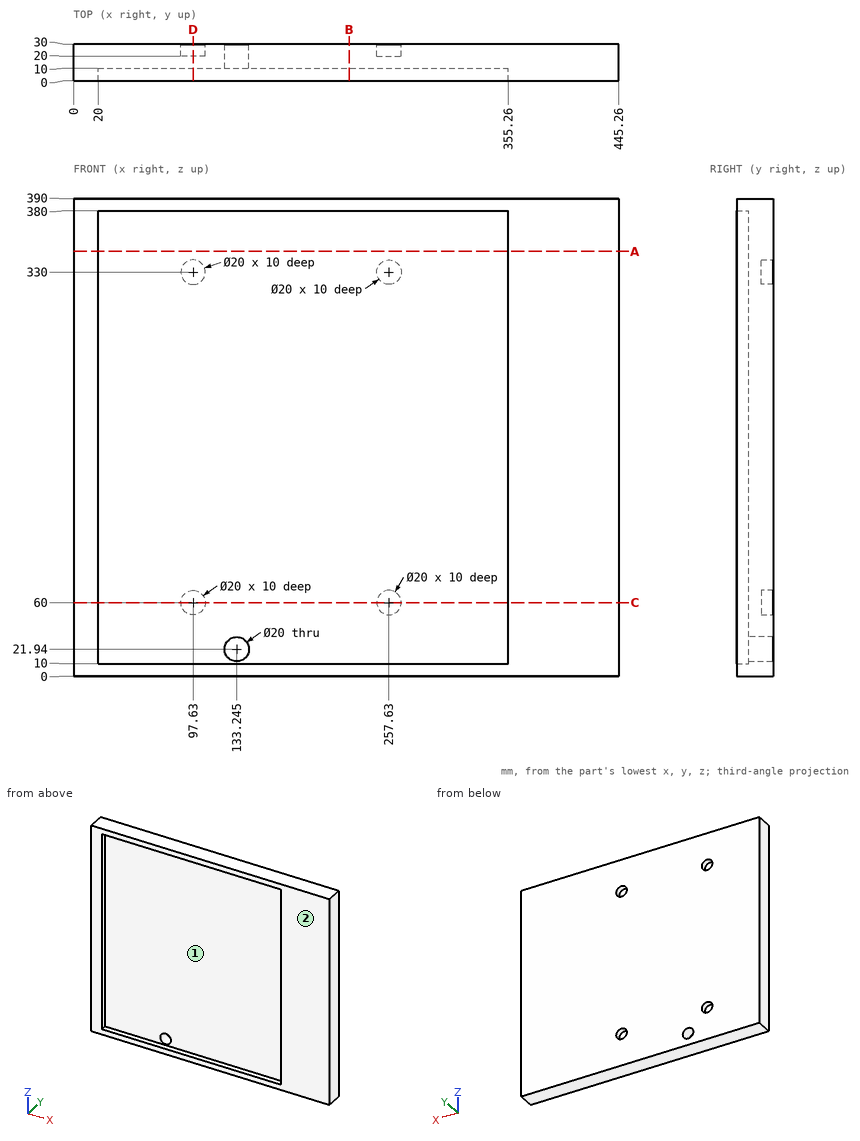
Geometry check sheet. Reference: drawing and pictorial views, mm from the part's lowest x, y, z. A direction names the side the tool comes from. Coordinates: 2 decimals unless noted, no trailing zeros. Write each loop counter-clockwise with the first axis right and the second up, starting at its lowest first coordinate (ties: lowest second). Pieces come first, ordered by that corner, then holes. Notation, with made-up numbers: M 21.5,28.5 L 60.5,28.5 A6 ccw 60.5,33.5 Z; hole C 86.5,10.5 d10. An arc over 180 degrees is marked long. Write item = value, one per line. Start each with the question number.
1. Sectioned sample at A-A (z = 347). Record the cut outline in (x, y), then the cut area to 3 significant figures.
2. Sectioned sample at B-B (x = 225). Record the cut outline in (y, z).
3. Tool access check on the marked faces 1 and 2. Record the directions out of +Z, -Z, +X, -X, +Y, -Y that give a thin tool (end or side, any length) a straight path to the whole face; none if there is none.
4. Thickness scan on probe 1 along X at (y, z) = (26.75, 60); probe 2 along Z at (x, y) = (69, 3.25); probe 3 along X at (y, z) = (2.25, 173). Record the ranges inside material, lowest first.
5. Go/stop test with flat-tipped pins: pin 1 (11 mm diameter, centred on x = 270, y = 5.5, fed in from -Z); pin 2 (12 mm diameter, centred on x = 257.63, z = 60, fed in from +Y); pin 3 (1 mm diameter, centred on x = 235, z = 172, fed in from -Y). Record where each tip stops, or that it passes through.
6. Sectioned sample at D-D (x = 97.63). Record the cut outline in (y, z), then the cut area to 3 significant figures.
7. Sectioned sample at C-C (z = 60). Record the cut outline in (x, y).
The answers:
q1.outline = M 0,0 L 20,0 L 20,10 L 355.26,10 L 355.26,0 L 445.26,0 L 445.26,30 L 0,30 Z
q1.area = 10,000 mm²
q2.outline = M 0,0 L 30,0 L 30,390 L 0,390 L 0,380 L 10,380 L 10,10 L 0,10 Z
q3.face_1 = -Y
q3.face_2 = +Z, -Z, +X, -X, -Y
q4.probe_1 = 0 to 87.63, 107.63 to 247.63, 267.63 to 445.26
q4.probe_2 = 0 to 10, 380 to 390
q4.probe_3 = 0 to 20, 355.26 to 445.26
q5.pin_1 = 0
q5.pin_2 = 20
q5.pin_3 = 10
q6.outline = M 0,0 L 30,0 L 30,50 L 20,50 L 20,70 L 30,70 L 30,320 L 20,320 L 20,340 L 30,340 L 30,390 L 0,390 L 0,380 L 10,380 L 10,10 L 0,10 Z
q6.area = 7,600 mm²
q7.outline = M 0,0 L 20,0 L 20,10 L 355.26,10 L 355.26,0 L 445.26,0 L 445.26,30 L 267.63,30 L 267.63,20 L 247.63,20 L 247.63,30 L 107.63,30 L 107.63,20 L 87.63,20 L 87.63,30 L 0,30 Z
